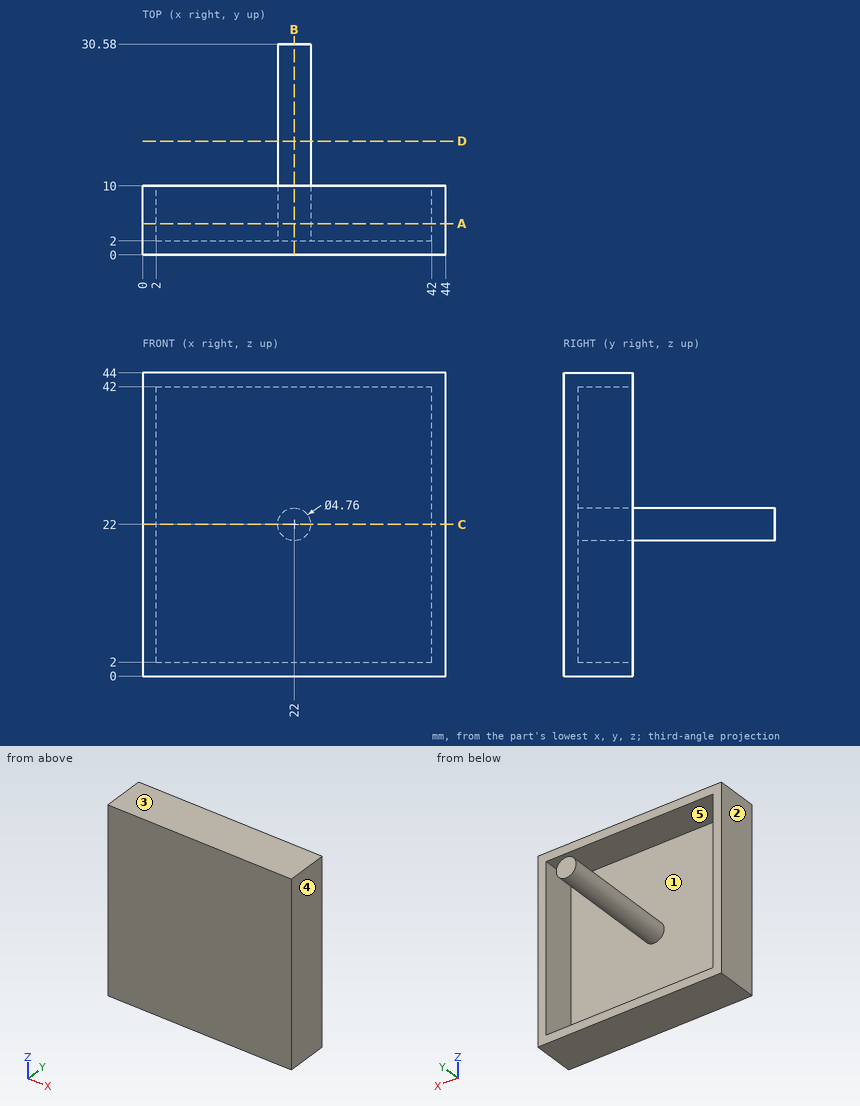
Study the drawing (mm; zero at the part's minimum x, y, z) and answer. A direction names the side the tool comes from. Round coordinates to 2 decimals unless told otherwise and drop trailing zeros. Order: outer loops, then holes, each group sorted by start corner. A loop starts at its lowest first (then second) coordinate and runs counter-clockwise, first axis right, second up. Notation, with made-up numbers: (59.25, 69) -> (65.25, 69) arc R22 cw to (65.25, 105) -> close; hole circle Ø4 at (-1, 84). An arc over 180 degrees is marked (long way). Write each question's results on one line, items separated by ' | '. Start each with the question number.
Q1. Which of the six approach directions +Z, -Z, +X, -X, +Y, -Y give full straight-line access (tool end or side, diameter ignored) to the marked faces 1 and 2?
Q2. Find section D-D (y = 16.5). Determine the outline of the cut face in (x, z).
Q3. Find section B-B (x = 22). Determine the outline of the cut face in (y, z).
Q4. The mould has two halves that part along Z. Classify the marked faces 3, 4 and 5: pulls with the +Z half, pulls with the -Z half, needs draft (parallel to the pull), parting line crosses it, or undercut.
Q5. Find section A-A (y = 4.5). Determine the outline of the cut face in (x, z), then the cut area to 3 significant figures.
Q6. Straight lines are drawn through the part: probe 1 along X at (y, z) = (8, 19); probe 2 along Z at (x, y) = (24, 5). For each, find the intervals that lie inside material, in ascending order. Write a range as from..to.
Q7. This flat-tipped pin is pushed along its axis until it touches: pin 1 (3 mm diameter, centred on x = 29.5, z = 29, fed in from +Y). Where does it stop, or does it pass through?
Q8. Find section C-C (z = 22). Determine the outline of the cut face in (x, y).
Worked answers:
1) face 1: +Y | face 2: +Z, -Z, -X, +Y, -Y
2) outline: circle Ø4.76 at (22, 22)
3) outline: (0, 0) -> (10, 0) -> (10, 2) -> (2, 2) -> (2, 19.62) -> (30.58, 19.62) -> (30.58, 24.38) -> (2, 24.38) -> (2, 42) -> (10, 42) -> (10, 44) -> (0, 44) -> close
4) face 3: pulls with the +Z half | face 4: needs draft | face 5: undercut
5) outline: (0, 0) -> (44, 0) -> (44, 44) -> (0, 44) -> close; circle Ø4.76 at (22, 22); hole (2, 2) -> (42, 2) -> (42, 42) -> (2, 42) -> close | area: 354 mm2
6) probe 1: x = 0..2, 42..44 | probe 2: z = 0..2, 20.71..23.29, 42..44
7) pin 1: stops at y = 2
8) outline: (0, 0) -> (44, 0) -> (44, 10) -> (42, 10) -> (42, 2) -> (24.38, 2) -> (24.38, 30.58) -> (19.62, 30.58) -> (19.62, 2) -> (2, 2) -> (2, 10) -> (0, 10) -> close
